```python
from build123d import *

# Parameters (mm, degrees)
SKETCH_1_W             = 80
SKETCH_1_H             = 40
EXTRUDE_1_DEPTH        = 5
SKETCH_2_W             = 10
SKETCH_2_H             = 30.1
CUT_EXTRUDE_1_DEPTH    = 2.1
PATTERN_LINEAR_1_COUNT = 6
PATTERN_LINEAR_1_PITCH = 13.33
EXTRUDE_2_DEPTH        = 80
CHAMFER_1_SIZE         = 6.1


with BuildPart() as part:
    # Эскиз1 → Бобышка-Вытянуть1 (new body)
    with BuildSketch(Plane(origin=(0, 0, 0), x_dir=(1, 0, 0), z_dir=(0, 1, 0))):
        Rectangle(SKETCH_1_W, SKETCH_1_H)
    extrude(amount=EXTRUDE_1_DEPTH)

    # Эскиз2 → Вырез-Вытянуть1 (cut)
    with BuildSketch(Plane(origin=(0, 5, 0), x_dir=(1, 0, 0), z_dir=(0, 1, 0))):
        with Locations((-33.34, 0)):
            Rectangle(SKETCH_2_W, SKETCH_2_H)
    cut_extrude_1 = extrude(amount=-CUT_EXTRUDE_1_DEPTH, mode=Mode.SUBTRACT)

    # Линейный массив1: Вырез-Вытянуть1 ×6
    with Locations(*[(i * PATTERN_LINEAR_1_PITCH, 0, 0) for i in range(1, PATTERN_LINEAR_1_COUNT)]):
        add(cut_extrude_1, mode=Mode.SUBTRACT)

    # Эскиз3 → Бобышка-Вытянуть2 (add)
    with BuildSketch(Plane.ZY.offset(40)):
        Polygon((-13.07, 0), (-13.07, -2), (-15.45, -2), (-15.45, -3.44), (-12.79, -6.1), (-7.21, -6.1), (-4.55, -3.44), (-4.55, -2), (-7.02, -2), (-7.02, 0), align=None)
        Polygon((7.02, 0), (13.07, 0), (13.07, -2), (15.45, -2), (15.45, -3.44), (12.79, -6.1), (7.21, -6.1), (4.55, -3.44), (4.55, -2), (7.02, -2), align=None)
    extrude(amount=-EXTRUDE_2_DEPTH)

    # Фаска1
    chamfer_1_edges = [part.edges().sort_by_distance(p)[0] for p in [
        (40, -6.1, 10),
        (-40, -6.1, 10),
        (40, -6.1, -10),
        (-40, -6.1, -10),
    ]]
    chamfer(chamfer_1_edges, length=CHAMFER_1_SIZE)


solid = part.part
```
Part model, mm, in its own coordinate system. A direction names the side the tool comes from. Round coordinates to 2 decimals unless told otherwise and drop trailing zeros. Loops run counter-clockwise (first coordinate to the right, second up) from the corner with the lowest first, then second, coordinate; pieces in that order, holes last.
Item 1: Cut at C-C, the plane z = 0.5. Give the cut face in (x, y), then the cut area to 3 significant figures.
Item 2: Drop flat-ended pins along their axis: P1, Ø12, axis at x = 24, z = 12.5, coming from the +Y side; P2, Ø3, axis at x = -18, z = -6.5, coming from the +Y side; P3, Ø3, axis at x = 1, z = 2.5, coming from the -Y side; P4, Ø1.2, axis at x = 11, y = -2.5, coming from the -Z side. Give the stop position or say it passes through.
Item 3: Cut at B-B, the plane y = 4. Give the cut face in (x, z).
Item 4: Mould opens along Y. For faces 1 (the face through (-1.68, 4, 0)), 2 (the face through (-1, -1, -7.02)), 3 (the face through (0, -6.1, -10)) say: +Y half, -Y half, draft (parallel to the pull), parting line (faces both ways), or undercut.
Item 5: 3-axis set-ups, long thin cutter, end or side, ignore diameter. For faces 4 (the face through (-0.51, -4.79, -5.9)), 5 (the face through (-1, 0, -17)), 6 (the face through (28.31, 4, 0)): which of +Z, -Z, +X, -X, +Y, -Y reach the whole face in a straight line?
Item 6: Cut at A-A, the plane y = -1.25. Give the cut face in (x, z), then the cut area to 3 significant figures.
Item 7: Cut at D-D, the plane x = 21.5. Give the cut face in (y, z).
Item 8: Drill centre lines: line 1 (Z direction, x = -2, y = 3); line 2 (Z direction, x = -35.5, y = -0.25); line 3 (Y direction, x = -29, z = -15.5). Where is each one in solid material? Low to high.
A:
1. outline: (-40, 0) - (40, 0) - (40, 5) - (38.31, 5) - (38.31, 2.9) - (28.31, 2.9) - (28.31, 5) - (24.98, 5) - (24.98, 2.9) - (14.98, 2.9) - (14.98, 5) - (11.65, 5) - (11.65, 2.9) - (1.65, 2.9) - (1.65, 5) - (-1.68, 5) - (-1.68, 2.9) - (-11.68, 2.9) - (-11.68, 5) - (-15.01, 5) - (-15.01, 2.9) - (-25.01, 2.9) - (-25.01, 5) - (-28.34, 5) - (-28.34, 2.9) - (-38.34, 2.9) - (-38.34, 5) - (-40, 5) - close
1. area: 274 mm2
2. P1: stops at y = 5
2. P2: stops at y = 2.9
2. P3: stops at y = 0
2. P4: stops at z = -15.45
3. outline: (-40, -20) - (40, -20) - (40, 20) - (-40, 20) - close; hole (-38.34, -15.05) - (-28.34, -15.05) - (-28.34, 15.05) - (-38.34, 15.05) - close; hole (-25.01, -15.05) - (-15.01, -15.05) - (-15.01, 15.05) - (-25.01, 15.05) - close; hole (-11.68, -15.05) - (-1.68, -15.05) - (-1.68, 15.05) - (-11.68, 15.05) - close; hole (1.65, -15.05) - (11.65, -15.05) - (11.65, 15.05) - (1.65, 15.05) - close; hole (14.98, -15.05) - (24.98, -15.05) - (24.98, 15.05) - (14.98, 15.05) - close; hole (28.31, -15.05) - (38.31, -15.05) - (38.31, 15.05) - (28.31, 15.05) - close
4. face 1: draft
4. face 2: undercut
4. face 3: -Y half
5. face 4: +X, -X, -Y
5. face 5: -Z, +X, -X
5. face 6: +Y
6. outline: (-38.75, -13.07) - (38.75, -13.07) - (38.75, -7.02) - (-38.75, -7.02) - close; (-38.75, 7.02) - (38.75, 7.02) - (38.75, 13.07) - (-38.75, 13.07) - close
6. area: 938 mm2
7. outline: (-6.1, -12.79) - (-3.44, -15.45) - (-2, -15.45) - (-2, -13.07) - (0, -13.07) - (0, -20) - (5, -20) - (5, -15.05) - (2.9, -15.05) - (2.9, 15.05) - (5, 15.05) - (5, 20) - (0, 20) - (0, 13.07) - (-2, 13.07) - (-2, 15.45) - (-3.44, 15.45) - (-6.1, 12.79) - (-6.1, 7.21) - (-3.44, 4.55) - (-2, 4.55) - (-2, 7.02) - (0, 7.02) - (0, -7.02) - (-2, -7.02) - (-2, -4.55) - (-3.44, -4.55) - (-6.1, -7.21) - close
8. line 1: z = -20 to -15.05, 15.05 to 20
8. line 2: z = -13.07 to -7.02, 7.02 to 13.07
8. line 3: y = 0 to 5
